```python
from build123d import *

# Parameters (mm, degrees)
SKETCH1_W           = 5
SKETCH1_H           = 60
BOSS_EXTRUDE1_DEPTH = 270
CUT_EXTRUDE1_REACH  = 273.708
SKETCH2_R           = 7.5
SKETCH2_R_2         = 10


with BuildPart() as part:
    # Sketch1 → Boss-Extrude1 (new body)
    with BuildSketch(Plane.XY):
        Rectangle(SKETCH1_W, SKETCH1_H)
    extrude(amount=BOSS_EXTRUDE1_DEPTH)

    # Sketch2 → Cut-Extrude1 (cut, up to next)
    with BuildSketch(Plane(origin=(2.5, 0, 0), x_dir=(0, 0, -1), z_dir=(1, 0, 0)), mode=Mode.PRIVATE) as cut_extrude1_sk1:
        with Locations((-60, 0)):
            Circle(SKETCH2_R)
    cut_extrude1_tool1 = extrude(cut_extrude1_sk1.sketch, amount=-CUT_EXTRUDE1_REACH, mode=Mode.PRIVATE) & part.part
    # Sketch2 → Cut-Extrude1 (cut, up to next)
    with BuildSketch(Plane(origin=(2.5, 0, 0), x_dir=(0, 0, -1), z_dir=(1, 0, 0)), mode=Mode.PRIVATE) as cut_extrude1_sk2:
        with Locations((-210, 0)):
            Circle(SKETCH2_R)
    cut_extrude1_tool2 = extrude(cut_extrude1_sk2.sketch, amount=-CUT_EXTRUDE1_REACH, mode=Mode.PRIVATE) & part.part
    # Sketch2 → Cut-Extrude1 (cut, up to next)
    with BuildSketch(Plane(origin=(2.5, 0, 0), x_dir=(0, 0, -1), z_dir=(1, 0, 0)), mode=Mode.PRIVATE) as cut_extrude1_sk3:
        with Locations((-250, 15)):
            Circle(SKETCH2_R_2)
    cut_extrude1_tool3 = extrude(cut_extrude1_sk3.sketch, amount=-CUT_EXTRUDE1_REACH, mode=Mode.PRIVATE) & part.part
    # Sketch2 → Cut-Extrude1 (cut, up to next)
    with BuildSketch(Plane(origin=(2.5, 0, 0), x_dir=(0, 0, -1), z_dir=(1, 0, 0)), mode=Mode.PRIVATE) as cut_extrude1_sk4:
        with Locations((-20, 15)):
            Circle(SKETCH2_R_2)
    cut_extrude1_tool4 = extrude(cut_extrude1_sk4.sketch, amount=-CUT_EXTRUDE1_REACH, mode=Mode.PRIVATE) & part.part
    add(cut_extrude1_tool1.solids().sort_by_distance((2.5, 0, 60))[0], mode=Mode.SUBTRACT)
    add(cut_extrude1_tool2.solids().sort_by_distance((2.5, 0, 210))[0], mode=Mode.SUBTRACT)
    add(cut_extrude1_tool3.solids().sort_by_distance((2.5, 15, 250))[0], mode=Mode.SUBTRACT)
    add(cut_extrude1_tool4.solids().sort_by_distance((2.5, 15, 20))[0], mode=Mode.SUBTRACT)


solid = part.part
```
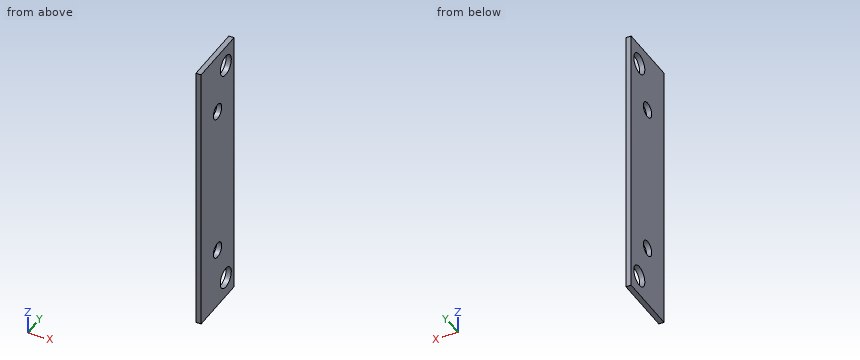
Source: CAD feature listing. Evaluate the final solid. Frame: model axes, mm. Coordinates: 2 decimals unless noted, no trailing zeros. Loops run counter-clockwise (first coordinate to the right, second up) from the corner with the lowest first, then second, coordinate; pieces in that order, holes last. Notation, with made-up numbers: (27.5, 45) -> (82.5, 45) arc R16 cw to (82.5, 61) -> close; hole circle Ø11 at (41, 4). An arc over 180 degrees is marked (long way). One line per item, written item: value. Start each with the question number.
Q1. Line query: line 1 along Y through (x, z) = (0.7, 210); line 2 along Y through (x, z) = (0.3, 250); line 3 along Z through (x, y) = (-1.25, -2.5). Output: solid intervals per line, ascending.
Q2. Section query B-B, the plane z = 20. Return the cut outline in (x, y).
Q3. Section query A-A, the plane y = 0. Return the cut outline in (x, z), and give its area (3 significant figures).
Q4. Section query C-C, the plane x = -0.4. Return the cut outline in (y, z), and give its area (3 significant figures).
Q5. Contact query for a flat-ended pin moving along its axis: P1, Ø12, axis at y = 15, z = 250, coming from the -X side. Output: stop coordinate, or through.
Q6. Section query D-D, the plane y = 15. Return the cut outline in (x, z).
Results:
1. line 1: -30 to -7.5, 7.5 to 30
1. line 2: -30 to 5, 25 to 30
1. line 3: 0 to 52.93, 67.07 to 202.93, 217.07 to 270
2. outline: (-2.5, -30) -> (2.5, -30) -> (2.5, 5) -> (-2.5, 5) -> close; (-2.5, 25) -> (2.5, 25) -> (2.5, 30) -> (-2.5, 30) -> close
3. outline: (-2.5, 0) -> (2.5, 0) -> (2.5, 52.5) -> (-2.5, 52.5) -> close; (-2.5, 67.5) -> (2.5, 67.5) -> (2.5, 202.5) -> (-2.5, 202.5) -> close; (-2.5, 217.5) -> (2.5, 217.5) -> (2.5, 270) -> (-2.5, 270) -> close
3. area: 1,200 mm^2
4. outline: (-30, 0) -> (30, 0) -> (30, 270) -> (-30, 270) -> close; hole circle Ø15 at (0, 60); hole circle Ø15 at (0, 210); hole circle Ø20 at (15, 20); hole circle Ø20 at (15, 250)
4. area: 15,200 mm^2
5. P1: through
6. outline: (-2.5, 0) -> (2.5, 0) -> (2.5, 10) -> (-2.5, 10) -> close; (-2.5, 30) -> (2.5, 30) -> (2.5, 240) -> (-2.5, 240) -> close; (-2.5, 260) -> (2.5, 260) -> (2.5, 270) -> (-2.5, 270) -> close
